Geometry: final body of the model. Coordinates: model frame, mm. Face numbers are marked on the shaded views. A direction names the side the tool comes from. Round coordinates to 2 decimals unless told otherwise and drop trailing zeros. Write each loop counter-clockwise with the first axis right and the second up, starting at its lowest first coordinate (ties: lowest second). Pieces come first, ordered by that corner, then holes. Notation, with made-up numbers: (10, 63) -> (46, 63) arc R22 ccw to (46, 82) -> close; hole circle Ø10 at (75.25, -3.75). An arc over 180 degrees is marked (long way). One line per item, written item: value. Start each with the question number.
from build123d import *

# Parameters (mm, degrees)
F1_DEPTH = 50.8
F2_DEPTH = 19.05
F3_DEPTH = 19.05
F5_R     = 5.08
F6_R     = 5.08
F7_DEPTH = 12.7


with BuildPart() as f1:
    # F0 (on Front) → F1 (new body, symmetric)
    with BuildSketch(Plane.XZ):
        Polygon((-60.4666993022, 30.4462667555), (-60.4666993022, -30.4462667555), (60.4666993022, -30.4462667555), (60.4666993022, 30.4462667555), (41.3047336042, 30.4462667555), (27.3347329348, 30.4462667555), align=None)
    extrude(amount=F1_DEPTH, both=True)

    # F0 (on Front) → F2 (join, symmetric)
    with BuildSketch(Plane.XZ):
        with BuildLine():
            Line((27.3347329348, 50.0340685248), (27.3347329348, 30.4462667555))
            Line((27.3347329348, 30.4462667555), (41.3047336042, 30.4462667555))
            Line((41.3047336042, 30.4462667555), (41.3047336042, 50.0340685248))
            ThreePointArc((41.3047336042, 50.0340685248), (46.8065044858, 64.3122336797), (60.4666993022, 71.2067648895))
            Line((60.4666993022, 71.2067648895), (60.4666993022, 85.2186777329))
            ThreePointArc((60.4666993022, 85.2186777329), (36.9213956127, 74.1985254838), (27.3347329348, 50.0340685248))
        make_face()
    extrude(amount=F2_DEPTH, both=True)

    # F0 (on Front) → F3 (join, symmetric)
    with BuildSketch(Plane.XZ):
        with BuildLine():
            ThreePointArc((62.5829263954, 85.2822619854), (61.5243353427, 85.2663623363), (60.4666993022, 85.2186777329))
            Line((60.4666993022, 85.2186777329), (60.4666993022, 71.2067648895))
            ThreePointArc((60.4666993022, 71.2067648895), (61.5234988842, 71.2858708439), (62.5829263954, 71.312261316))
            Line((62.5829263954, 71.312261316), (75.3704831004, 71.312261316))
            Line((75.3704831004, 71.312261316), (75.3704831004, 85.2822619854))
            Line((75.3704831004, 85.2822619854), (62.5829263954, 85.2822619854))
        make_face()
    extrude(amount=F3_DEPTH, both=True)

    # F0 (on Front) → F4 (revolve)
    with BuildSketch(Plane.XZ):
        Polygon((90.2742668986, 93.8937179744), (75.3704831004, 93.8937179744), (75.3704831004, 85.2822619854), (75.3704831004, 71.312261316), (75.3704831004, 59.8279722035), (90.2742668986, 59.8279722035), align=None)
    revolve(axis=Axis((75.3704831004, 0, 76.860845089), (0, 0, 1)))

    # F5
    f5_edges = [f1.edges().sort_by_distance(p)[0] for p in [
        (60.466699, -50.8, 0),
        (60.466699, 50.8, 0),
        (-60.466699, 50.8, 0),
        (-60.466699, -50.8, 0),
    ]]
    fillet(f5_edges, radius=F5_R)

    # F6
    f6_edges = [f1.edges().sort_by_distance(p)[0] for p in [
        (60.466699, 0, 93.893718),
        (60.466699, 0, 59.827972),
    ]]
    fillet(f6_edges, radius=F6_R)

    # F0 (on Front) → F7 (join, symmetric)
    with BuildSketch(Plane.XZ):
        with BuildLine():
            add(Edge.make_bspline(
                [(-60.4666993022, 30.4462667555), (-27.2727292031, 30.4462667555), (0, 62.5284537673), (27.3347329348, 50.0340685248)],
                knots=[0, 0, 0, 0, 89.9598437139, 89.9598437139, 89.9598437139, 89.9598437139], degree=3))
            Line((-60.4666993022, 30.4462667555), (27.3347329348, 30.4462667555))
            Line((27.3347329348, 30.4462667555), (27.3347329348, 50.0340685248))
        make_face()
    extrude(amount=F7_DEPTH, both=True)


solid = f1.part
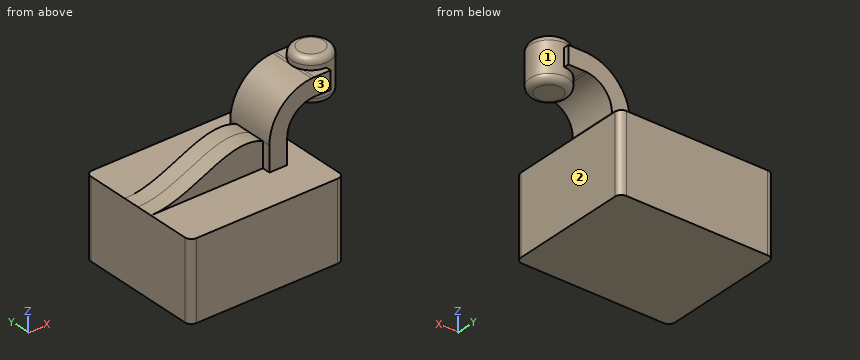
(1) Pin query (flat end, axial travel): pin 1 (6 mm diameter, centred on y = 7.5, z = 43, fed in from +X); pin 2 (1.9 mm diameter, centred on y = 17, z = 39, fed in from -X); pin 3 (1.5 mm diameter, centred on x = 45.5, y = -6, fed in from +Z); pin 4 (8 mm diameter, centred on x = -25, z = 32.5, fed in from -Y). Return the tip coordinate at first contact, or that it passes through.
(2) Section query B-B (x = 47). Output: boundary loops of the cut face in (y, z).
(3) Section query A-A (z = 25). Output: boundary loops of the cut face in (x, y), and give its area (3 significant figures).
(4) Set-up query: the marked faces 1, 2 and 3. Return all of +Z, -Z, +X, -X, +Y, -Y with unobstructed straight access to the full face (end or side cutting, diameter ignored); none if empty.
(5) Section query D-D (z = 75.5). Output: boundary loops of the cut face in (x, y).
(6) Section query C-C (y = -26). Output: boundary loops of the cut face in (x, z).
(7) Line query: probe 1 along Z at (x, y) = (38, 34); probe 2 along X at (y, z) = (16, -14); probe 3 along Y at (x, z) = (-38, 33). Output: solid intervals per line, ascending.
Results list:
1. pin 1: stops at x = 41.3
1. pin 2: stops at x = 27.33
1. pin 3: stops at z = 81.27
1. pin 4: stops at y = -50.8
2. outline: (-50.8, -30.45) -> (50.8, -30.45) -> (50.8, 30.45) -> (-50.8, 30.45) -> close; (-19.05, 64.52) -> (19.05, 64.52) -> (19.05, 81.65) -> (-19.05, 81.65) -> close
3. outline: (-60.47, -45.72) arc R5.08 ccw to (-55.39, -50.8) -> (55.39, -50.8) arc R5.08 ccw to (60.47, -45.72) -> (60.47, 45.72) arc R5.08 ccw to (55.39, 50.8) -> (-55.39, 50.8) arc R5.08 ccw to (-60.47, 45.72) -> close
3. area: 12,300 mm^2
4. face 1: none
4. face 2: -Z, +X, +Y, -Y
4. face 3: +Z, +X, -X, -Y
5. outline: (38.21, -19.05) -> (75.37, -19.05) -> (75.37, -14.9) arc R14.9 ccw to (75.37, 14.9) -> (75.37, 19.05) -> (38.21, 19.05) -> close
6. outline: (-60.47, -30.45) -> (60.47, -30.45) -> (60.47, 30.45) -> (-60.47, 30.45) -> close
7. probe 1: z = -30.45 to 30.45
7. probe 2: x = -60.47 to 60.47
7. probe 3: y = -12.7 to 12.7
